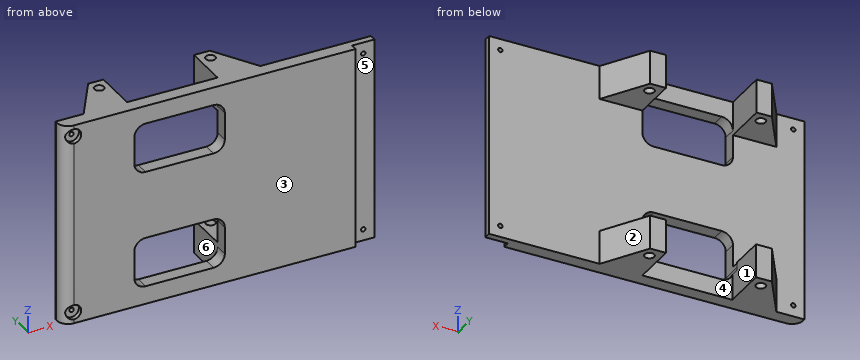
```python
from build123d import *

# Parameters (mm, degrees)
SKIZZE1_W                             = 140
SKIZZE1_H                             = 90
AUFSATZ_LINEAR_AUSTRAGEN1_DEPTH       = 6
SKIZZE2_W                             = 10
SKIZZE2_H                             = 90
SCHNITT_LINEAR_AUSTRAGEN1_DEPTH       = 3
SKIZZE3_W                             = 7.06
SKIZZE3_H                             = 25.7
SKIZZE3_R                             = 2.1
AUFSATZ_LINEAR_AUSTRAGEN2_DEPTH       = 15
AUFSATZ_LINEAR_START                  = -15
SKIZZE4_W                             = 6.783859635
SKIZZE4_H                             = 25.7
SKIZZE4_R                             = 2.1
SKIZZE4_W_2                           = 7.06
AUFSATZ_LINEAR_AUSTRAGEN3_DEPTH       = 15
VERRUNDUNG1_R                         = 5
SCHNITT_LINEAR_AUSTRAGEN2_DEPTH       = 10
SKIZZE6_R                             = 0.975
SCHNITT_LINEAR_AUSTRAGEN3_DEPTH       = 10
SKIZZE7_R                             = 3.25
SCHNITT_LINEAR_AUSTRAGEN4_DEPTH       = 2
AUFSATZ_LINEAR_START_2                = -90
AUFSATZ_LINEAR_AUSTRAGEN4_OUTLINE_R   = 2.15
AUFSATZ_LINEAR_AUSTRAGEN4_OUTLINE_R_2 = 2.1
AUFSATZ_LINEAR_AUSTRAGEN4_DEPTH       = 90
AUFSATZ_LINEAR_AUSTRAGEN4_2_DEPTH     = 15
AUFSATZ_LINEAR_AUSTRAGEN5_DEPTH       = 15
AUFSATZ_LINEAR_AUSTRAGEN6_DEPTH       = 15


# Read off the part's stored shape, not the designer's step: Aufsatz-Linear austragen4
with BuildPart() as part:
    # Skizze1 → Aufsatz-Linear austragen1 (new body)
    with BuildSketch(Plane(origin=(0, 0, 0), x_dir=(1, 0, 0), z_dir=(0, 1, 0))):
        with Locations((70, 45)):
            Rectangle(SKIZZE1_W, SKIZZE1_H)
    extrude(amount=AUFSATZ_LINEAR_AUSTRAGEN1_DEPTH)

    # Skizze2 → Schnitt-Linear austragen1 (cut)
    with BuildSketch(Plane.XZ):
        with Locations((135, -45)):
            Rectangle(SKIZZE2_W, SKIZZE2_H)
    extrude(amount=-SCHNITT_LINEAR_AUSTRAGEN1_DEPTH, mode=Mode.SUBTRACT)

    # Skizze3 → Aufsatz-Linear austragen2 (add)
    # profile 1 of 2: a face of its own
    with BuildSketch(Plane(origin=(0, 0, -90), x_dir=(-1, 0, 0), z_dir=(0, 0, -1))):
        with Locations((-75.49, 12.85)):
            Rectangle(SKIZZE3_W, SKIZZE3_H)
        with Locations((-76.72, 20.78)):
            Circle(SKIZZE3_R, mode=Mode.SUBTRACT)
    # profile 2 of 2: a face of its own
    with BuildSketch(Plane(origin=(0, 0, -90), x_dir=(-1, 0, 0), z_dir=(0, 0, -1))):
        with Locations((-28.53, 12.85)):
            Rectangle(SKIZZE3_W, SKIZZE3_H)
        with Locations((-27.3, 20.78)):
            Circle(SKIZZE3_R, mode=Mode.SUBTRACT)
    extrude(amount=-AUFSATZ_LINEAR_AUSTRAGEN2_DEPTH)

    # Skizze4 → Aufsatz-Linear austragen3 (add)
    # profile 1 of 2: a face of its own
    with BuildSketch(Plane.XY.offset(AUFSATZ_LINEAR_START)):
        with Locations((28.391929817, 12.85)):
            Rectangle(SKIZZE4_W, SKIZZE4_H)
        with Locations(Location((27.3, 20.78, 0), (0, 0, 180))):
            Circle(SKIZZE4_R, mode=Mode.SUBTRACT)
    # profile 2 of 2: a face of its own
    with BuildSketch(Plane.XY.offset(AUFSATZ_LINEAR_START)):
        with Locations((75.49, 12.85)):
            Rectangle(SKIZZE4_W_2, SKIZZE4_H)
        with Locations(Location((76.72, 20.78, 0), (0, 0, 180))):
            Circle(SKIZZE4_R, mode=Mode.SUBTRACT)
    extrude(amount=AUFSATZ_LINEAR_AUSTRAGEN3_DEPTH)

    # Verrundung1
    verrundung1_edges = [part.edges().sort_by_distance(p)[0] for p in [
        (0, 0, -45),
    ]]
    fillet(verrundung1_edges, radius=VERRUNDUNG1_R)

    # Skizze5 → Schnitt-Linear austragen2 (cut)
    with BuildSketch(Plane(origin=(0, 0, 0), x_dir=(-1, 0, 0), z_dir=(0, -1, 0))):
        with BuildLine():
            Line((-36.783859635, 8), (-66.96, 8))
            ThreePointArc((-66.96, 8), (-70.495533906, 9.464466094), (-71.96, 13))
            Line((-71.96, 13), (-71.96, 25))
            ThreePointArc((-71.96, 25), (-70.495533906, 28.535533906), (-66.96, 30))
            Line((-66.96, 30), (-36.783859635, 30))
            ThreePointArc((-36.783859635, 30), (-33.248325729, 28.535533906), (-31.783859635, 25))
            Line((-31.783859635, 25), (-31.783859635, 13))
            ThreePointArc((-31.783859635, 13), (-33.248325729, 9.464466094), (-36.783859635, 8))
        make_face()
        with BuildLine():
            Line((-36.783859635, 82), (-66.96, 82))
            ThreePointArc((-66.96, 82), (-70.495533906, 80.535533906), (-71.96, 77))
            Line((-71.96, 77), (-71.96, 65))
            ThreePointArc((-71.96, 65), (-70.495533906, 61.464466094), (-66.96, 60))
            Line((-66.96, 60), (-36.783859635, 60))
            ThreePointArc((-36.783859635, 60), (-33.248325729, 61.464466094), (-31.783859635, 65))
            Line((-31.783859635, 65), (-31.783859635, 77))
            ThreePointArc((-31.783859635, 77), (-33.248325729, 80.535533906), (-36.783859635, 82))
        make_face()
    extrude(amount=-SCHNITT_LINEAR_AUSTRAGEN2_DEPTH, mode=Mode.SUBTRACT)

    # Skizze6 → Schnitt-Linear austragen3 (cut)
    with BuildSketch(Plane.XZ):
        with Locations(Location((135, -5, 0), (0, 0, 270))):
            Circle(SKIZZE6_R)
        with Locations(Location((5, -85, 0), (0, 0, 270))):
            Circle(SKIZZE6_R)
        with Locations(Location((135, -85, 0), (0, 0, 270))):
            Circle(SKIZZE6_R)
        with Locations(Location((5, -5, 0), (0, 0, 270))):
            Circle(SKIZZE6_R)
    extrude(amount=-SCHNITT_LINEAR_AUSTRAGEN3_DEPTH, mode=Mode.SUBTRACT)

    # Skizze7 → Schnitt-Linear austragen4 (cut)
    with BuildSketch(Plane.XZ):
        with Locations(Location((5, -5, 0), (0, 0, 270))):
            Circle(SKIZZE7_R)
        with Locations(Location((5, -85, 0), (0, 0, 270))):
            Circle(SKIZZE7_R)
    extrude(amount=-SCHNITT_LINEAR_AUSTRAGEN4_DEPTH, mode=Mode.SUBTRACT)

    # Aufsatz-Linear austragen4 outline → Aufsatz-Linear austragen4 (cut)
    # profile 1 of 2: a face of its own
    with BuildSketch(Plane(origin=(0, 0, -90), x_dir=(-1, 0, 0), z_dir=(0, 0, -1)).offset(AUFSATZ_LINEAR_START_2)):
        with Locations((-76.72, 20.78)):
            Circle(AUFSATZ_LINEAR_AUSTRAGEN4_OUTLINE_R)
        with Locations((-76.72, 20.78)):
            Circle(AUFSATZ_LINEAR_AUSTRAGEN4_OUTLINE_R_2, mode=Mode.SUBTRACT)
    # profile 2 of 2: a face of its own
    with BuildSketch(Plane(origin=(0, 0, -90), x_dir=(-1, 0, 0), z_dir=(0, 0, -1)).offset(AUFSATZ_LINEAR_START_2)):
        with Locations((-27.3, 20.78)):
            Circle(AUFSATZ_LINEAR_AUSTRAGEN4_OUTLINE_R)
        with Locations((-27.3, 20.78)):
            Circle(AUFSATZ_LINEAR_AUSTRAGEN4_OUTLINE_R_2, mode=Mode.SUBTRACT)
    extrude(amount=AUFSATZ_LINEAR_AUSTRAGEN4_DEPTH, mode=Mode.SUBTRACT)

    # Aufsatz-Linear austragen4 2 outline → Aufsatz-Linear austragen4 2 (add)
    with BuildSketch(Plane(origin=(0, 0, -90), x_dir=(-1, 0, 0), z_dir=(0, 0, -1)).offset(AUFSATZ_LINEAR_START)):
        Polygon((-79.02, 6), (-79.02, 25.7), (-90.903397377, 6), align=None)
    extrude(amount=AUFSATZ_LINEAR_AUSTRAGEN4_2_DEPTH)

    # Skizze10 → Aufsatz-Linear austragen5 (add)
    with BuildSketch(Plane(origin=(0, 0, -90), x_dir=(-1, 0, 0), z_dir=(0, 0, -1))):
        Polygon((-25, 25.7), (-12.5, 6), (-25, 6), align=None)
    extrude(amount=-AUFSATZ_LINEAR_AUSTRAGEN5_DEPTH)

    # Skizze11 → Aufsatz-Linear austragen6 (add)
    with BuildSketch(Plane.XY):
        Polygon((25, 25.7), (12.5, 6), (25, 6), align=None)
        Polygon((79.02, 25.7), (79.02, 6), (90.903397377, 6), align=None)
    extrude(amount=-AUFSATZ_LINEAR_AUSTRAGEN6_DEPTH)


solid = part.part
```
Geometry check sheet. Reference: the model listing, model coordinates, mm. Face numbers are marked on the shaded views. A direction names the side the tool comes from. Give positions to 0.01 mm unless a question says otherwise; leave off trailing zeros. Order: outer loops, then holes, each group sorted by start corner. A loop starts at its lowest first (then second) coordinate and runs counter-clockwise, first axis right, second up.
1. Section check B-B, the plane x = 27.3. Enter the section's corners in (y, z), and give its area (3 significant figures).
2. Thickness scan on L1, parallel to X at y = 5.1, z = -85 (3 decimals); L2, parallel to X at y = 20.78, z = -9.25; L3, parallel to Z at x = 32, y = 14.25. Record the ranges inside material, lowest first.
3. Gauge pin test, flat ends, axial feed: pin 1 Ø5 at (x, z) = (5.5, -85) entering from -Y; pin 2 Ø5.5 at (x, y) = (76.72, 20.78) entering from -Z; pin 3 Ø12.5 at (y, z) = (18.5, -15) entering from -X; pin 4 Ø4.5 at (y, z) = (11.5, -83) entering from +X. Record the tip position at first contact, or that the pin passes through.
4. Release check for a two-part mould opening along X. For the marked faces 1, 2 and 3 record: pulls with the +X half, pulls with the -X half, needs draft (parallel to the pull), parting line crosses it, or undercut.
5. Section check A-A, the plane z = -66.5. Enter the section's corners in (x, y), and give its area (3 significant figures).
6. Section check C-C, the plane y = 20.78. Give the number of separate pieces and of enclosed holes in the cut face, and give its area (3 significant figures).
7. Section check D-D, the plane z = -47.5. Enter the section's corners in (x, y), and give its area (3 significant figures).
8. Access from +Z, -Z, +X, -X, +Y, -Y to the whole of each face (thin tool, end or side, straight path). Record for the marked faces 4, 5 and 6.
Values follow:
1. outline: (0, -90) - (18.63, -90) - (18.63, -75) - (6, -75) - (6, -15) - (18.63, -15) - (18.63, 0) - (0, 0) - close; (22.93, -90) - (25.7, -90) - (25.7, -75) - (22.93, -75) - close; (22.93, -15) - (25.7, -15) - (25.7, 0) - (22.93, 0) - close
1. area: 1,000 mm2
2. L1: x = 0 to 4.025, 5.975 to 134.025, 135.975 to 140
2. L2: x = 21.88 to 25.15, 29.45 to 31.78, 71.96 to 74.57, 78.87 to 81.99
2. L3: z = -90 to -75
3. pin 1: stops at y = 2
3. pin 2: stops at z = -90
3. pin 3: stops at x = 16.47
3. pin 4: stops at x = 88.94
4. face 1: undercut
4. face 2: pulls with the +X half
4. face 3: needs draft
5. outline: (0, 5) arc R5 ccw to (5, 0) - (31.78, 0) - (31.78, 6) - (0, 6) - close; (71.96, 0) - (130, 0) - (130, 3) - (140, 3) - (140, 6) - (71.96, 6) - close
5. area: 564 mm2
6. separate pieces: 8
6. enclosed holes: 0
6. area: 344 mm2
7. outline: (0, 5) arc R5 ccw to (5, 0) - (130, 0) - (130, 3) - (140, 3) - (140, 6) - (0, 6) - close
7. area: 805 mm2
8. face 4: +Z, -Z, +Y
8. face 5: +Z, -Z, +X, -Y
8. face 6: +Y
